Here's how the part is built. I have some questions about the finished solid (model axes, mm). Round coordinates to 2 decimals unless told otherwise and drop trailing zeros. Write each loop counter-clockwise with the first axis right and the second up, starting at its lowest first coordinate (ties: lowest second). Pieces come first, ordered by that corner, then holes. Notation, with made-up numbers: (-38.5, 48.5) - (2.5, 48.5) arc R17 ccw to (2.5, 61.5) - close; hole circle Ø3 at (56, 7). An arc over 180 degrees is marked (long way). One line per item, written item: value. Start each with the question number.
Item 1: Imagine slicing it at A-A, the plane y = 0. Please give me the cut outline in (x, z), then the cut area to 3 significant figures.
Item 2: For P1, Ø4, axis at y = 2.5, z = 61.5, coming from the -X side; P2, Ø8, axis at x = -5, y = -2, coming from the +Z side; P3, Ø1, axis at x = -3, z = 131, coming from the -Y side, each with a flat end and sliding along its axis, tell me the tip position at first contact or that it passes through.
Item 3: Imagine slicing it at D-D, the plane z = 102.5. Please give me the cut outline in (x, y), then the cut area to 3 significant figures.
Item 4: Imagine slicing it at C-C, the plane x = 0. Count the separate pieces of the cut face and the enclosed holes in it, then the cut area to 3 significant figures.
Item 5: If I drill on line 1 (Z direction, x = 0, y = 4.6); line 2 (X direction, y = -4.65, z = 0); line 3 (Z direction, x = 5, y = -3.5), over which ranges is the centre line in solid material (lowest first)?
Item 6: Imagine slicing it at B-B, the plane z = 231. Please give me the cut outline in (x, y) (3 decimals).
```python
from build123d import *

# Parameters (mm, degrees)
BOSS_EXTRUDE1_START             = -1
SKETCH2_R                       = 4
BOSS_EXTRUDE1_DEPTH             = 11
SKETCH3_R                       = 7.5
BOSS_EXTRUDE2_DEPTH             = 194
CHAMFER1_SIZE                   = 2
CHAMFER2_SIZE                   = 2
BOSS_EXTRUDE3_REACH             = 233.278
BOSS_EXTRUDE3_END_RADIUS        = 8.5
SKETCH5_R                       = 4
BOSS_EXTRUDE3_DIRECTION_2_DEPTH = 10


with BuildPart() as part:
    # Sketch1 → Revolve2 (revolve)
    with BuildSketch(Plane.XY):
        with BuildLine():
            Line((6.148407421, 4.295007123), (6.148407421, 5))
            Line((6.148407421, 5), (8.5, 5))
            Line((8.5, 5), (8.5, -5))
            Line((8.5, -5), (6.148407421, -5))
            Line((6.148407421, -5), (6.148407421, -4.295007123))
            ThreePointArc((6.148407421, -4.295007123), (7.5, 0), (6.148407421, 4.295007123))
        make_face()
    revolve(axis=Axis((0, -1000, 0), (0, 1, 0)))

    # Sketch2 → Boss-Extrude1 (add)
    with BuildSketch(Plane.XY.offset(8.5).offset(BOSS_EXTRUDE1_START)):
        Circle(SKETCH2_R)
    extrude(amount=BOSS_EXTRUDE1_DEPTH)

    # Sketch3 → Boss-Extrude2 (add)
    with BuildSketch(Plane.XY.offset(18.5)):
        with Locations(Location((0, 0, 0), (0, 0, 180))):
            Circle(SKETCH3_R)
    extrude(amount=BOSS_EXTRUDE2_DEPTH)

    # Chamfer1
    chamfer1_edges = [part.edges().sort_by_distance(p)[0] for p in [
        (7.5, 0, 18.5),
    ]]
    chamfer(chamfer1_edges, length=CHAMFER1_SIZE)

    # Chamfer2
    chamfer2_edges = [part.edges().sort_by_distance(p)[0] for p in [
        (7.5, 0, 212.5),
    ]]
    chamfer(chamfer2_edges, length=CHAMFER2_SIZE)



with BuildPart() as body_2:
    # Sketch4 → Revolve3 (revolve)
    with BuildSketch(Plane.XY.offset(231)):
        with BuildLine():
            Line((6.148407421, 5), (6.148407421, 4.295007123))
            ThreePointArc((6.148407421, 4.295007123), (7.5, 0), (6.148407421, -4.295007123))
            Line((6.148407421, -4.295007123), (6.148407421, -5))
            Line((6.148407421, -5), (8.5, -5))
            Line((8.5, -5), (8.5, 5))
            Line((8.5, 5), (6.148407421, 5))
        make_face()
    revolve(axis=Axis((0, -1000, 231), (0, 1, 0)))


with BuildPart() as part_1:
    add(part.part)

    add(body_2.part)  # Boss-Extrude3 merges body 2
    # Boss-Extrude3: up to this cylinder (the profile starts outside it)
    boss_extrude3_end = Plane(origin=(0, 0, 231), z_dir=(0, -1, 0)) * Cylinder(BOSS_EXTRUDE3_END_RADIUS, 484.556, mode=Mode.PRIVATE)
    # Sketch5 → Boss-Extrude3 (add, up to the surface)
    with BuildSketch(Plane(origin=(0, 0, 222.5), x_dir=(-1, 0, 0), z_dir=(0, 0, -1)), mode=Mode.PRIVATE) as boss_extrude3_sk1:
        with Locations(Location((0, 0, 0), (0, 0, 180))):
            Circle(SKETCH5_R)
    boss_extrude3_tool1 = extrude(boss_extrude3_sk1.sketch, amount=-BOSS_EXTRUDE3_REACH, mode=Mode.PRIVATE) - boss_extrude3_end
    add(boss_extrude3_tool1.solids().sort_by_distance((0, 0, 222.5))[0])
    add(boss_extrude3_tool1.solids().sort_by_distance((0, 0, 222.5))[1])

    # Sketch5 → Boss-Extrude3 direction 2 (add)
    with BuildSketch(Plane(origin=(0, 0, 222.5), x_dir=(-1, 0, 0), z_dir=(0, 0, -1))):
        with Locations(Location((0, 0, 0), (0, 0, 180))):
            Circle(SKETCH5_R)
    extrude(amount=BOSS_EXTRUDE3_DIRECTION_2_DEPTH)


solid = part_1.part
```
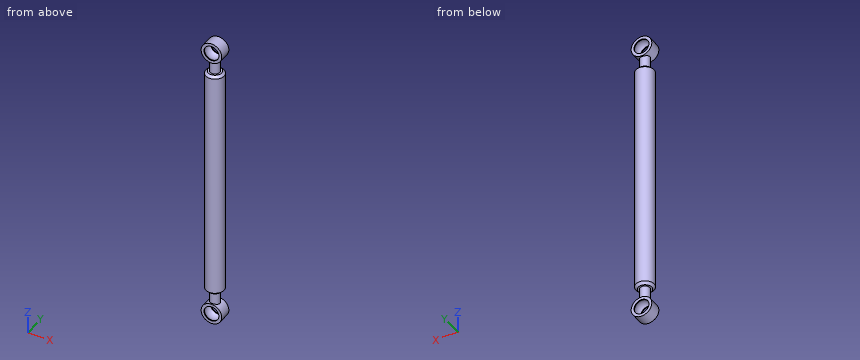
Values follow:
1. outline: (-7.5, 20.5) - (-5.5, 18.5) - (-4, 18.5) - (-4, 7.5) arc R8.5 ccw (long way) to (4, 7.5) - (4, 18.5) - (5.5, 18.5) - (7.5, 20.5) - (7.5, 210.5) - (5.5, 212.5) - (4, 212.5) - (4, 223.5) arc R8.5 ccw (long way) to (-4, 223.5) - (-4, 212.5) - (-5.5, 212.5) - (-7.5, 210.5) - close; hole circle Ø15 at (0, 0); hole circle Ø15 at (0, 231)
1. area: 3,170 mm^2
2. P1: stops at x = -7.48
2. P2: stops at z = 239.44
2. P3: stops at y = -7.07
3. outline: circle Ø15 at (0, 0)
3. area: 177 mm^2
4. separate pieces: 3
4. enclosed holes: 0
4. area: 3,120 mm^2
5. line 1: z = -8.5 to -6.15, 6.15 to 8.5, 18.5 to 212.5, 222.5 to 224.85, 237.15 to 239.5
5. line 2: x = -8.5 to -6.15, 6.15 to 8.5
5. line 3: z = -6.87 to -4.36, 4.36 to 6.87, 19.1 to 211.9, 224.13 to 226.64, 235.36 to 237.87
6. outline: (-8.5, -5) - (-6.148, -5) - (-6.148, -4.295) arc R7.5 cw to (-6.148, 4.295) - (-6.148, 5) - (-8.5, 5) - close; (6.148, -5) - (8.5, -5) - (8.5, 5) - (6.148, 5) - (6.148, 4.295) arc R7.5 cw to (6.148, -4.295) - close
